Here's how the part is built. I have some questions about the finished solid (model axes, mm). A direction names the side the tool comes from. Give positions to 0.01 mm unless a question says otherwise; leave off trailing zeros. Order: outer loops, then holes, each group sorted by start corner. A loop starts at its lowest first (then second) coordinate and runs counter-clockwise, first axis right, second up. Notation, with made-up numbers: M 23.25,84 L 50.25,84 A21 ccw 50.25,107 Z; hole C -2,66.25 d6. An arc over 180 degrees is marked long. One line per item, written item: value. Start each with the question number.
from build123d import *

# Parameters (mm, degrees)
F1_DEPTH  = 7
F4_DEPTH  = 54.8
F5_R      = 9.5
F6_DEPTH  = 42
F8_R      = 4.5
F9_DEPTH  = 25
F10_R     = 4.5
F11_DEPTH = 10.5
F12_R     = 4.5
F15_R     = 1.25
F16_DEPTH = 10
F18_DEPTH = 3
F2_R      = 2.5
F19_DEPTH = 12


with BuildPart() as f1:
    # F0 (on Top) → F1 (new body)
    with BuildSketch(Plane.XY):
        Polygon((-25, -25), (0, -25), (25, -25), (25, 25), (-25, 25), align=None)
    extrude(amount=F1_DEPTH)

    # F3 (on face) → F4 (join)
    with BuildSketch(Plane.XY):
        Polygon((-25, -10), (0, -10), (25, -10), (25, 5), (-25, 5), align=None)
    extrude(amount=-F4_DEPTH)

    # F5 (on face) → F6 (cut)
    with BuildSketch(Plane(origin=(0, 0, -54.8), x_dir=(1, 0, 0), z_dir=(0, 0, -1))):
        with Locations((0, 10)):
            Circle(F5_R)
    extrude(amount=-F6_DEPTH, mode=Mode.SUBTRACT)

    # F8 (on offset) → F9 (cut)
    with BuildSketch(Plane.XY.offset(-4.5)):
        with Locations((0, -10)):
            Circle(F8_R)
    extrude(amount=-F9_DEPTH, mode=Mode.SUBTRACT)

    # F10 (on face) → F11 (cut)
    with BuildSketch(Plane.XZ.offset(25)):
        Circle(F10_R)
    extrude(amount=-F11_DEPTH, mode=Mode.SUBTRACT)

    # F14: sweep along a path in F13
    with BuildLine(Plane.YZ) as f14_path:
        ThreePointArc((-10, -4.5), (-11.318019, -1.318019), (-14.5, 0))
    # F12 (on offset) → F14 (sweep, cut)
    with BuildSketch(Plane.XY.offset(-4.5)):
        with Locations((0, -10)):
            Circle(F12_R)
    sweep(path=f14_path.line, mode=Mode.SUBTRACT)

    # F15 (on face) → F16 (cut)
    with BuildSketch(Plane.XZ.offset(10)):
        with Locations((15, -35)):
            Circle(F15_R)
        with Locations((-15, -35)):
            Circle(F15_R)
    extrude(amount=-F16_DEPTH, mode=Mode.SUBTRACT)

    # F17 (on face) → F18 (join)
    with BuildSketch(Plane(origin=(0, 0, -12.8), x_dir=(1, 0, 0), z_dir=(0, 0, -1))):
        with BuildLine():
            Line((-2.015418, 14.023443), (-2.015418, 19.130202))
            ThreePointArc((-2.015418, 19.130202), (0, 0.65), (2.015418, 19.130202))
            Line((2.015418, 19.130202), (2.015418, 14.023443))
            ThreePointArc((2.015418, 14.023443), (0, 5.5), (-2.015418, 14.023443))
        make_face()
    extrude(amount=-F18_DEPTH)

    # F2 (on face) → F19 (cut)
    with BuildSketch(Plane.XY.offset(7)):
        with Locations((0, 4)):
            Circle(F2_R)
    extrude(amount=-F19_DEPTH, mode=Mode.SUBTRACT)


solid = f1.part
Item 1: Please list where these lines run through material, in increasing order: probe 1 along Z at (x, y) = (-15, -2); probe 2 along X at (y, z) = (4, -2.25); probe 3 along Z at (x, y) = (-16.5, -11). Write a range as [from, to].
Item 2: Will these pins go through, and if not, where does the flat tip stop? P1, Ø10, axis at x = -1, z = -16.5, coming from the -Y side; P2, Ø1.5, axis at x = 15, z = -35, coming from the +Y side; P3, Ø3.5, axis at y = -16.5, z = -12, coming from the +X side; P4, Ø3, axis at x = -0.5, y = 2.5, coming from the +Z side.
Item 3: I want a section at A-A on x = -19.5. Write out the boundary of the cut face in (y, z).
Item 4: For faces 1 (the face through (-16.25, -5.07, -34.95)), 2 (the face through (-7.233, -15.924, -11.321)), 3 (the face through (-0.209, -0.502, -34.094)), which set-ups out of +Z, -Z, +X, -X, +Y, -Y let a thin tool reach every point of the face, with its end or its side?
Item 5: We'd pull the mould along Y, two halves only. Please class faces 4 (the face through (7.34, -15.79, -11.32)), 5 (the face through (0, 5, -27)), 6 (the face through (-0.54, 1.56, 1.08)), 7 (the face through (25, -2, -19)): +Y half, -Y half, draft (parallel to the pull), parting line (faces both ways), or undercut.
Item 6: I want a section at B-B on z = -35. Write out the boundary of the cut face in (x, y).
Item 7: I want a section at D-D on x = -7.5. Write out the boundary of the cut face in (y, z).
Item 8: I want a section at C-C on y = 12. Write out the boundary of the cut face in (x, z).
Answer below:
1. probe 1: z = [-54.8, -36.25], [-33.75, 7]
1. probe 2: x = [-25, -2.5], [2.5, 25]
1. probe 3: z = [0, 7]
2. P1: stops at y = -19.13
2. P2: stops at y = 5
2. P3: stops at x = 8.05
2. P4: stops at z = 7
3. outline: M -25,0 L -10,0 L -10,-54.8 L 5,-54.8 L 5,0 L 25,0 L 25,7 L -25,7 Z
4. face 1: -Y
4. face 2: -Z, -X, -Y
4. face 3: -Z, -Y
5. face 4: -Y half
5. face 5: +Y half
5. face 6: undercut
5. face 7: draft
6. outline: M -25,-10 L -16.25,-10 L -16.25,0 L -13.75,0 L -13.75,-10 L -9.5,-10 A9.5 cw 9.5,-10 L 13.75,-10 L 13.75,0 L 16.25,0 L 16.25,-10 L 25,-10 L 25,5 L -25,5 Z
7. outline: M -25,0 L -10,0 L -10,-9.8 L -15.58,-9.8 L -15.58,-12.8 L -4.17,-12.8 L -4.17,-54.8 L 5,-54.8 L 5,0 L 25,0 L 25,7 L -25,7 Z
8. outline: M -25,0 L 25,0 L 25,7 L -25,7 Z
